from build123d import *

# Parameters (mm, degrees)
SKETCH1_R           = 6
BOSS_EXTRUDE1_DEPTH = 4


with BuildPart() as part:
    # Sketch1 → Boss-Extrude1 (new body)
    with BuildSketch(Plane.XY):
        with BuildLine():
            Line((0, 0), (170, 0))
            ThreePointArc((170, 0), (180.12069735, 5.5524047), (180.875693444, 17.071419141))
            Line((180.875693444, 17.071419141), (153.405506431, 75.981425298))
            ThreePointArc((153.405506431, 75.981425298), (137.458393846, 81.785699602), (131.654119542, 65.838587016))
            Line((131.654119542, 65.838587016), (138.559595063, 51.029746973))
            ThreePointArc((138.559595063, 51.029746973), (137.36418458, 32.791307441), (121.339747109, 24))
            Line((121.339747109, 24), (0, 24))
            ThreePointArc((0, 24), (-12, 12), (0, 0))
        make_face()
        with Locations((142.529812987, 70.910006157)):
            Circle(SKETCH1_R, mode=Mode.SUBTRACT)
        with BuildLine():
            Line((0, 18), (100, 18))
            ThreePointArc((100, 18), (106, 12), (100, 6))
            Line((100, 6), (0, 6))
            ThreePointArc((0, 6), (-6, 12), (0, 18))
        make_face(mode=Mode.SUBTRACT)
        Polygon((170, 18.92820323), (164, 15.464101615), (164, 8.535898385), (170, 5.07179677), (176, 8.535898385), (176, 15.464101615), align=None, mode=Mode.SUBTRACT)
    extrude(amount=BOSS_EXTRUDE1_DEPTH)


solid = part.part
Source: CAD feature listing. Evaluate the final solid. Frame: model axes, mm. A direction names the side the tool comes from. Give positions to 0.01 mm unless a question says otherwise; leave off trailing zeros. Write each loop counter-clockwise with the first axis right and the second up, starting at its lowest first coordinate (ties: lowest second). Pieces come first, ordered by that corner, then holes. Notation, with made-up numbers: M 65.25,59 L 118.25,59 A23 cw 118.25,93 Z; hole C 86,-36 d1. An arc over 180 degrees is marked long. Answer as a JSON object with one key per item and string values.
Q1. Ray query, line 1 along Y through (x, z) = (-0.5, 1.75); line 2 along Y through (x, z) = (142, 0.6); line 3 along Y through (x, z) = (116.5, 2.2). Return the intervals inside material, ascending.
Geometry check:
{"line 1": "y = 0.01 to 6.02, 17.98 to 23.99", "line 2": "y = 0 to 64.93, 76.89 to 82.9", "line 3": "y = 0 to 24"}
Q2. Access query for faces 1 (the face through (84, 0, 2)), 2 (the face through (120, 23, 0)), 3 (the face through (62, 24, 2)), 4 (the face through (135.059, 58.538, 1.972)), 5 (the face through (-6, 12, 2)). Directions: +Z, -Z, +X, -X, +Y, -Y. A direction counts if a zero-diameter tool reaches every point of the face in a straight line with its end or side. Return the directions, or none.
Geometry check:
{"face 1": "+Z, -Z, +X, -X, -Y", "face 2": "-Z, +X, -X, +Y, -Y", "face 3": "+Z, -Z, -X, +Y", "face 4": "+Z, -Z, -X", "face 5": "+Z, -Z"}
Q3. Cut plane B-B, the plane x = 77. Return the cut outline in (y, z), then the cut area to 3 significant figures.
Geometry check:
{"outline": "M 0,0 L 6,0 L 6,4 L 0,4 Z; M 18,0 L 24,0 L 24,4 L 18,4 Z", "area": "48.0 mm^2"}
Q4. Cut plane A-A, the plane y = 12. Return the cut outline in (x, z), then the cut area to 3 significant figures.
Geometry check:
{"outline": "M -12,0 L -6,0 L -6,4 L -12,4 Z; M 106,0 L 164,0 L 164,4 L 106,4 Z; M 176,0 L 182,0 L 182,4 L 176,4 Z", "area": "280 mm^2"}
Q5. Cut plane C-C, the plane z = 2.75. Return the cut outline in (x, y).
Geometry check:
{"outline": "M 0,0 L 170,0 A12 ccw 180.88,17.07 L 153.41,75.98 A12 ccw 131.65,65.84 L 138.56,51.03 A19 cw 121.34,24 L 0,24 A12 ccw Z; hole M 0,6 L 100,6 A6 ccw 100,18 L 0,18 A6 ccw Z; hole C 142.53,70.91 d12; hole M 164,8.54 L 170,5.07 L 176,8.54 L 176,15.46 L 170,18.93 L 164,15.46 Z"}
Q6. Contact query for flat-ended pins moving along their axis: P1, Ø2, axis at y = 11, z = 2.5, coming from the -X side; P2, Ø1, axis at x = 145, z = 3, coming from the +Y side; P3, Ø2, axis at x = 64, z = 2.5, coming from the +Y side; P4, Ø12, axis at x = 101.5, y = 35, coming from the -Z side. Output: stop coordinate, or through.
Geometry check:
{"P1": "stops at x = -12", "P2": "stops at y = 82.75", "P3": "stops at y = 24", "P4": "passes through"}
Q7. Cut plane D-D, the plane y = 73.5. Return the cut outline in (x, z), then the cut area to 3 significant figures.
Geometry check:
{"outline": "M 130.81,0 L 137.12,0 L 137.12,4 L 130.81,4 Z; M 147.94,0 L 154.56,0 L 154.56,4 L 147.94,4 Z", "area": "51.7 mm^2"}
Q8. Mould query, pull axis Y, two halves, no side actions, for faces 6 (the face through (51, 6, 2)), 7 (the face through (180.03, 5.41, 1.97)), 8 (the face through (120, 23, 4)), 9 (the face through (167.04, 17.22, 1.97)). Classes: +Y half, -Y half, draft (parallel to the pull), parting line (faces both ways), or undercut.
Geometry check:
{"face 6": "undercut", "face 7": "parting line", "face 8": "draft", "face 9": "undercut"}
